For this review, use the dimensioned drawing (mm, ordinates from the lowest corner) and the shaded views. A direction names the side the tool comes from. Round coordinates to 2 decimals unless told otherwise and drop trailing zeros. Loops run counter-clockwise (first coordinate to the right, second up) from the corner with the lowest first, then second, coordinate; pieces in that order, holes last.
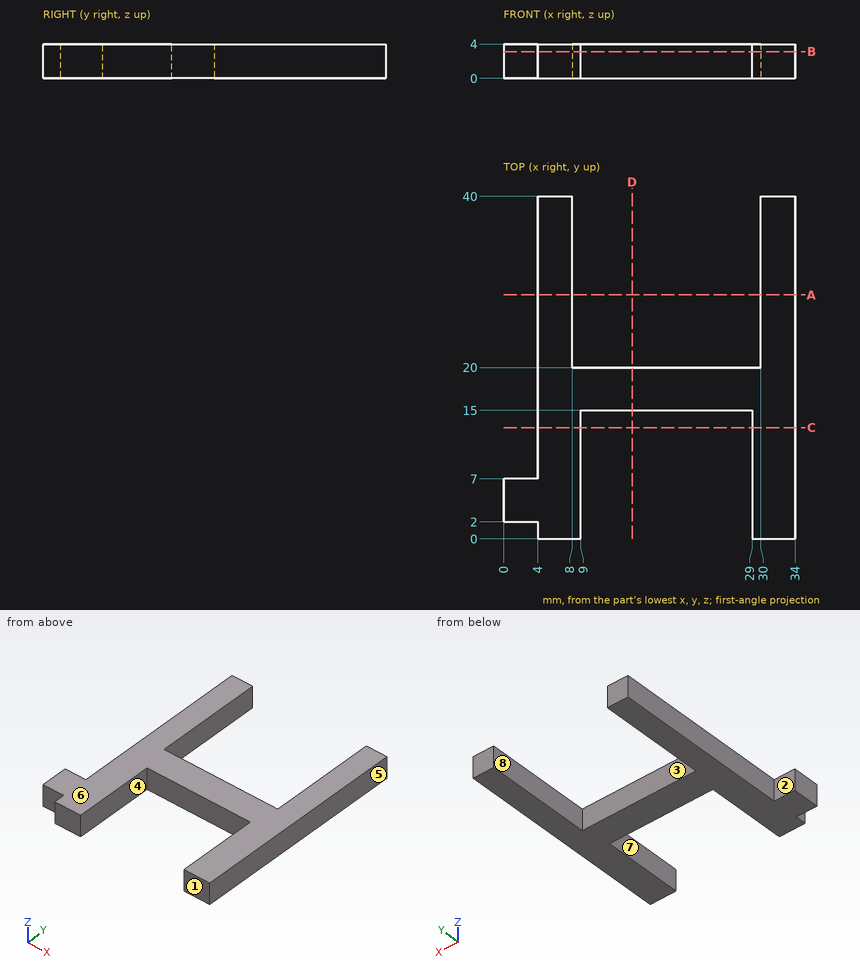
(1) Add section B-B (z = 3.1). Give the boundary of the cut face in (x, y).
(2) For L1, parallel to X at y = 6, z = 2.1; L2, parallel to X at y = 26.5, z = 1; L3, parallel to Y at x = 23, z = 0.55, list the stretches that pass through material, from the lowest coordinate up.
(3) Add section D-D (x = 15). Give the boundary of the cut face in (y, z), plus the area to 3 significant figures.
(4) Add section A-A (y = 28.5). Give the boundary of the cut face in (x, z).
(5) Insertion check: pin 1 Ø1.2 at (x, z) = (23.5, 1.5) entering from +Y; pin 2 Ø2 at (x, z) = (1.5, 1) entering from +Y; pin 3 Ø2 at (y, z) = (30.5, 2.5) entering from -X. Each pin has a flat end and moves straight along its axis. Give the tip position at first contact, or say it passes through.
(6) The part is to be moulded in two halves that separate along X. For the marked faces 5, 6, 7 and 8, say which applies: pulls with the +X half, pulls with the -X half, needs draft (parallel to the pull), parting line crosses it, or undercut.
(7) For the marked faces 1, 2, 3 and 4, list the 3-axis set-ups (+Z, -Z, +X, -X, +Y, -Y) from which the entire face can be reached by the end or side of a thin tool; tool diameter is ignored.
(8) Add section C-C (y = 13). Give the boundary of the cut face in (x, z).
Outcome:
1. outline: (0, 2) - (4, 2) - (4, 0) - (9, 0) - (9, 15) - (29, 15) - (29, 0) - (34, 0) - (34, 40) - (30, 40) - (30, 20) - (8, 20) - (8, 40) - (4, 40) - (4, 7) - (0, 7) - close
2. L1: x = 0 to 9, 29 to 34
2. L2: x = 4 to 8, 30 to 34
2. L3: y = 15 to 20
3. outline: (15, 0) - (20, 0) - (20, 4) - (15, 4) - close
3. area: 20.0 mm2
4. outline: (4, 0) - (8, 0) - (8, 4) - (4, 4) - close; (30, 0) - (34, 0) - (34, 4) - (30, 4) - close
5. pin 1: stops at y = 20
5. pin 2: stops at y = 7
5. pin 3: stops at x = 4
6. face 5: pulls with the +X half
6. face 6: needs draft
6. face 7: undercut
6. face 8: undercut
7. face 1: +Z, -Z, +X, -X, -Y
7. face 2: +Z, -Z, -X, +Y
7. face 3: +Z, -Z, +Y
7. face 4: +Z, -Z, -Y
8. outline: (4, 0) - (9, 0) - (9, 4) - (4, 4) - close; (29, 0) - (34, 0) - (34, 4) - (29, 4) - close
